Here's the drawing with two shaded views (mm, measured from the low corner). I have some questions. A direction names the side the tool comes from. Round coordinates to 2 decimals unless told otherwise and drop trailing zeros. Loops run counter-clockwise (first coordinate to the right, second up) from the corner with the lowest first, then second, coordinate; pieces in that order, holes last. Notation, with made-up numbers: M -11,-15.5 L -1,-15.5 A35 ccw -1,17.5 Z; hole C -6.75,13.5 d8. An arc over 180 degrees is marked long. One line per item, written item: value. Start each with the question number.
Q1. Imagine slicing it at C-C (x = 49). Please give me the cut outline in (y, z).
Q2. Imagine slicing it at B-B (x = 119.5). Please give me the cut outline in (y, z).
Q3. Please list where these lines run through material, in increasing order: line 1 along X through (y, z) = (10, 107); line 2 along Y through (x, z) = (79, 106); line 3 along Y through (x, z) = (191, 61).
Q4. Which directions (+Z, -Z, +X, -X, +Y, -Y) give clear straight access to the entire face, cutting with the end or side of a thin tool? Please do the marked faces 1, 2 and 3.
Q5. I'm going to push flat-ended pins straight in: pin 1 Ø2 at (y, z) = (44.5, 87) entering from +X; pin 2 Ø21.5 at (y, z) = (26, 86) entering from -X; pin 3 Ø12 at (x, z) = (144, 82) entering from -Y. Where does each tip first touch, or does it pass through?
Q6. Imagine slicing it at A-A (z = 29). Please give me the cut outline in (x, y).
Q7. Imagine slicing it at D-D (y = 64). Please give me the cut outline in (x, z).
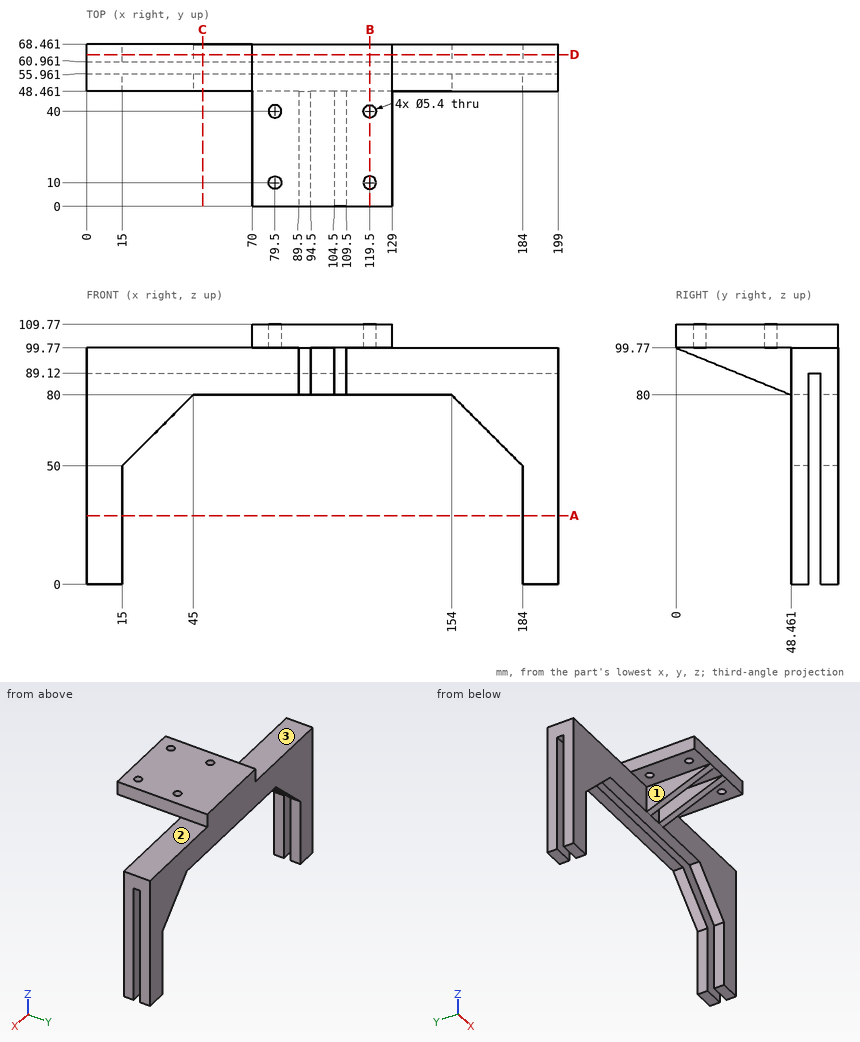
Report:
1. outline: M 48.46,80 L 55.96,80 L 55.96,89.12 L 60.96,89.12 L 60.96,80 L 68.46,80 L 68.46,99.77 L 48.46,99.77 Z
2. outline: M 0,99.77 L 7.3,99.77 L 7.3,109.77 L 0,109.77 Z; M 12.7,99.77 L 37.3,99.77 L 37.3,109.77 L 12.7,109.77 Z; M 42.7,99.77 L 48.46,99.77 L 48.46,80 L 55.96,80 L 55.96,89.12 L 60.96,89.12 L 60.96,80 L 68.46,80 L 68.46,109.77 L 42.7,109.77 Z
3. line 1: x = 70 to 76.8, 82.2 to 116.8, 122.2 to 129
3. line 2: y = 0 to 7.35, 12.65 to 37.35, 42.65 to 68.46
3. line 3: y = 48.46 to 55.96, 60.96 to 68.46
4. face 1: -Z, -X, -Y
4. face 2: +Z, +X, +Y, -Y
4. face 3: +Z, -X, +Y, -Y
5. pin 1: stops at x = 109.5
5. pin 2: stops at x = 89.5
5. pin 3: stops at y = 48.46
6. outline: M 0,48.46 L 15,48.46 L 15,55.96 L 0,55.96 Z; M 0,60.96 L 15,60.96 L 15,68.46 L 0,68.46 Z; M 184,48.46 L 199,48.46 L 199,55.96 L 184,55.96 Z; M 184,60.96 L 199,60.96 L 199,68.46 L 184,68.46 Z
7. outline: M 0,0 L 15,0 L 15,50 L 45,80 L 154,80 L 184,50 L 184,0 L 199,0 L 199,99.77 L 129,99.77 L 129,109.77 L 70,109.77 L 70,99.77 L 0,99.77 Z
